Geometry check sheet. Reference: drawing and pictorial views, mm from the part's lowest x, y, z. Round coordinates to 2 decimals unless told otherwise and drop trailing zeros. Write each loop counter-clockwise with the first axis right and the second up, starting at its lowest first coordinate (ties: lowest second). Pieces come first, ordered by that corner, then holes. Notation, with made-up numbers: M 30,6 L 45,6 A27 cw 45,40 Z; hole C 55.25,64.5 d6. An arc over 180 degrees is marked long. Put each result on its own line as item: value. Start each with the question number.
(1) Section check A-A on x = 15.5. Record the cut outline in (y, z).
(2) Mould release check, pull along Y, two halves, no side actions. Record for the marked faces 1, 2, 3 and 4: pulls with the +Y half, pulls with the -Y half, needs draft (parallel to the pull), parting line crosses it, or undercut.
(3) Section check D-D on y = 26. Record the cut outline in (x, z).
(4) Section check C-C on z = 1.6. Record the cut outline in (x, y), then the cut area to 3 significant figures.
(5) Material ranges on probe 1 along Y at (x, z) = (15.5, 1.25); probe 2 along X at (y, z) = (13, 0.4); probe 3 along Y at (x, z) = (19, 1.1), recorded low to high.
(6) Gauge pin test, flat end, axial feed: pin 1 (9.5 mm diameter, centred on x = 15.5, y = 15.5, fed in from -Z). Record the tip position at first contact, or that the pin passes through.
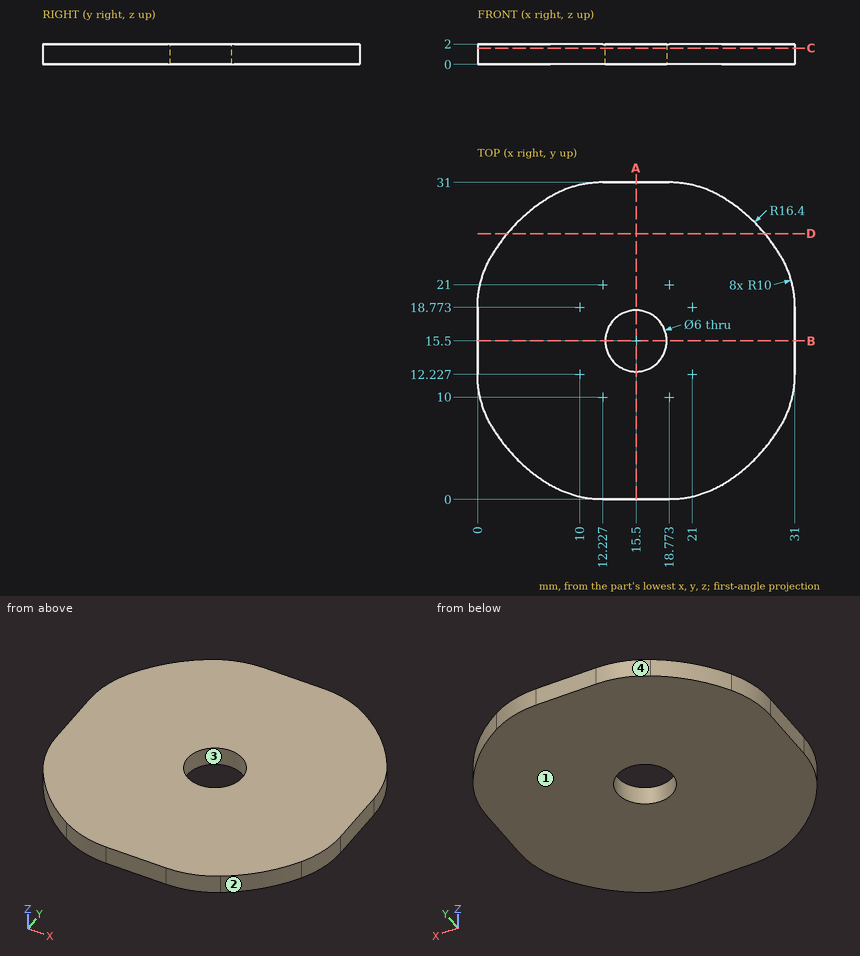
Answers follow:
1. outline: M 0,0 L 12.5,0 L 12.5,2 L 0,2 Z; M 18.5,0 L 31,0 L 31,2 L 18.5,2 Z
2. face 1: needs draft
2. face 2: pulls with the -Y half
2. face 3: undercut
2. face 4: pulls with the +Y half
3. outline: M 2.9,0 L 28.1,0 L 28.1,2 L 2.9,2 Z
4. outline: M 0,12.23 A10 ccw 1.41,7.11 A16.4 ccw 7.11,1.41 A10 ccw 12.23,0 L 18.77,0 A10 ccw 23.89,1.41 A16.4 ccw 29.59,7.11 A10 ccw 31,12.23 L 31,18.77 A10 ccw 29.59,23.89 A16.4 ccw 23.89,29.59 A10 ccw 18.77,31 L 12.23,31 A10 ccw 7.11,29.59 A16.4 ccw 1.41,23.89 A10 ccw 0,18.77 Z; hole C 15.5,15.5 d6
4. area: 788 mm^2
5. probe 1: y = 0 to 12.5, 18.5 to 31
5. probe 2: x = 0 to 13.84, 17.16 to 31
5. probe 3: y = 0 to 31
6. pin 1: stops at z = 0
